```python
from build123d import *

# Parameters (mm, degrees)
F0_R     = 7.9375
F1_DEPTH = 25.4
F2_W     = 6.35
F2_H     = 6.35
F3_DEPTH = 11.43
F4_W     = 5.588
F4_H     = 2.667
F5_DEPTH = 12.7


with BuildPart() as f1:
    # F0 (on Top) → F1 (new body)
    with BuildSketch(Plane.XY):
        Circle(F0_R)
    extrude(amount=F1_DEPTH)

    # F2 (on face) → F3 (cut)
    with BuildSketch(Plane.XY.offset(25.4)):
        Rectangle(F2_W, F2_H)
    extrude(amount=-F3_DEPTH, mode=Mode.SUBTRACT)

    # F4 (on face) → F5 (cut)
    with BuildSketch(Plane(origin=(0, 0, 0), x_dir=(1, 0, 0), z_dir=(0, 0, -1))):
        Rectangle(F4_W, F4_H)
    extrude(amount=-F5_DEPTH, mode=Mode.SUBTRACT)


solid = f1.part
```
Can you work these out from the model? Positions are in its coordinate system, mm. A direction names the side the tool comes from. Round coordinates to 2 decimals unless told otherwise and drop trailing zeros. Order: outer loops, then holes, each group sorted by start corner. A loop starts at its lowest first (then second) coordinate and runs counter-clockwise, first axis right, second up. Notation, with made-up numbers: (-13.5, 72.25) -> (22.5, 72.25) arc R20 cw to (22.5, 96.25) -> close; hole circle Ø5 at (18.5, 74.25). An arc over 180 degrees is marked (long way). Return JSON: item names as keys, results as strings. Group by question number.
1. Will these pins go through, and if not, where does the flat tip stop? pin 1 (7 mm diameter, centred on x = 0.5, z = 17.5, fed in from +Y); pin 2 (2 mm diameter, centred on x = -6, z = 7, fed in from -Y); pin 3 (5 mm diameter, centred on y = 3.5, z = 7, fed in from -X).
2. We'd pull the mould along X, two halves only. Please class faces 4 (the face through (0, 3.175, 20)), 5 (the face through (0, 0, 12.7)), 6 (the face through (0, -2, 0)), 7 (the face through (-1.72, -7.75, 12.52)): released by +X, released by -X, zero draft, split by the parting line, or undercut.
3. If we section it at A-A, the plane y = 0: Write out the boundary of the cut face in (x, z) (1 decimal).
4. If we section it at B-B, the plane z = 5.75: Write out the boundary of the cut face in (x, y) (1 decimal).
5. Which directions (+Z, -Z, +X, -X, +Y, -Y) give clear straight access to the entire face, cutting with the end or side of a thin tool? Please do faces 1 (the face through (3.4, 0.1, 25.4)), 2 (the face through (0, -3.175, 20)), 3 (the face through (0, -1.334, 6)).
6. I need wall thicknesses on line 1 (Z direction, x = -0.75, y = 1); line 2 (Y direction, x = 0.5, z = 18) (3 decimals); line 3 (X direction, y = -1, z = 4). Which ranges of each line are inside material? Lowest first, please. Write a range as [from, to].
7. If we section it at C-C, the plane x = 0: Write out the boundary of the cut face in (y, z) (1 decimal).
8. If we section it at D-D, the plane z = 22.25: Write out the boundary of the cut face in (x, y) (1 decimal).
Output values:
{
 "1": {"pin 1": "y = 7.94", "pin 2": "y = -6.16", "pin 3": "x = -7.87"},
 "2": {"face 4": "undercut", "face 5": "undercut", "face 6": "zero draft", "face 7": "split by the parting line"},
 "3": {"outline": "(-7.9, 0) -> (-2.8, 0) -> (-2.8, 12.7) -> (2.8, 12.7) -> (2.8, 0) -> (7.9, 0) -> (7.9, 25.4) -> (3.2, 25.4) -> (3.2, 14) -> (-3.2, 14) -> (-3.2, 25.4) -> (-7.9, 25.4) -> close"},
 "4": {"outline": "circle Ø15.9 at (0, 0); hole (-2.8, -1.3) -> (2.8, -1.3) -> (2.8, 1.3) -> (-2.8, 1.3) -> close"},
 "5": {"face 1": "+Z, +X, -X, +Y, -Y", "face 2": "+Z", "face 3": "-Z"},
 "6": {"line 1": "[12.7, 13.97]", "line 2": "[-7.922, -3.175], [3.175, 7.922]", "line 3": "[-7.87, -2.79], [2.79, 7.87]"},
 "7": {"outline": "(-7.9, 0) -> (-1.3, 0) -> (-1.3, 12.7) -> (1.3, 12.7) -> (1.3, 0) -> (7.9, 0) -> (7.9, 25.4) -> (3.2, 25.4) -> (3.2, 14) -> (-3.2, 14) -> (-3.2, 25.4) -> (-7.9, 25.4) -> close"},
 "8": {"outline": "circle Ø15.9 at (0, 0); hole (-3.2, -3.2) -> (3.2, -3.2) -> (3.2, 3.2) -> (-3.2, 3.2) -> close"}
}
